Part model, mm, in its own coordinate system. A direction names the side the tool comes from. Coordinates: 2 decimals unless noted, no trailing zeros. Write each loop counter-clockwise with the first axis right and the second up, starting at its lowest first coordinate (ties: lowest second). Pieces come first, ordered by that corner, then holes. Notation, with made-up numbers: M 15,44 L 42,44 A4 ccw 42,51 Z; hole C 12.5,-8.5 d5. An arc over 180 degrees is marked long. Use a Markdown table: item, result. Add a question column.
Q1. Slice it at B-B on y = 22.5. Write the cut outline in (x, z).
Q2. Mould opens along Y. For faces 4 (the flat face through (1.5, 26, 14.8)), 5 (the flat face through (19, 10, 15)), 6 (the flat face through (-9, 23, 17)) say: released by +Y, released by -Y, zero draft, split by the parting line, or undercut.
Q3. Slice it at A-A on z = 18. Write the cut outline in (x, y), then the cut area to 3 significant figures.
Q4. Slice it at C-C on x = 1. Write the cut outline in (y, z), then the cut area to 3 significant figures.
Q5. Pin check, flat tips, straight feed: pin 1 Ø6 at (x, z) = (16.5, 10) entering from -Y; pin 2 Ø1.5 at (x, z) = (18, 10.5) entering from +Y; pin 3 Ø8 at (y, z) = (3.5, 8) entering from +X. Stop position of each tip, or through.
Q6. Slice it at D-D on x = -20.5. Write the cut outline in (y, z).
Q7. Wall check: L1, parallel to Z at x = -17.5, y = 19.75; L2, parallel to X at y = 3.5, z = 1; L3, parallel to Y at x = 2, z = 19. Give the ranges that are in metal, low to high. Write a range as from..to.
Q8. Tool access for faces 1 (the flat face through (13, 5, 15)), 2 (the flat face through (17, 24, 5)), 3 (the flat face through (-13, 5, 15)): list every direction of +Z, -Z, +X, -X, +Y, -Y with a clear straight run to the whole face (end or side of a thin tool).
from build123d import *

# Parameters (mm, degrees)
EXTRUDE_1_DEPTH = 30
SKETCH_2_W      = 50
SKETCH_2_H      = 20
EXTRUDE_2_DEPTH = 5


with BuildPart() as part:
    # Эскиз1 → Бобышка-Вытянуть1 (new body)
    with BuildSketch(Plane.XY):
        Polygon((9, 17), (9, 23.5), (3, 23.5), (0, 18.5), (0, 0), (13, 0), (13, 10), (25, 10), (25, 17), align=None)
        Polygon((3, 23.5), (9, 23.5), (9, 30), (0, 30), (0, 28.5), align=None)
    extrude_1 = extrude(amount=EXTRUDE_1_DEPTH)

    # Зеркальное отражение1: Бобышка-Вытянуть1 across plane
    add(extrude_1.mirror(Plane(origin=(0, 0, 30), x_dir=(0, 0, 1), z_dir=(-1, 0, 0))))

    # Эскиз2 → Бобышка-Вытянуть2 (add)
    with BuildSketch(Plane(origin=(0, 0, 0), x_dir=(-1, 0, 0), z_dir=(0, 0, -1))):
        with Locations((0, 20)):
            Rectangle(SKETCH_2_W, SKETCH_2_H)
        Polygon((0, 28.5), (3, 23.5), (0, 18.5), (-3, 23.5), align=None, mode=Mode.SUBTRACT)
    extrude(amount=-EXTRUDE_2_DEPTH)


solid = part.part
Recorded:
| question | item | result |
|---|---|---|
| 1 | outline | M -25,0 L -2.4,0 L -2.4,30 L -9,30 L -9,5 L -25,5 Z; M 2.4,0 L 25,0 L 25,5 L 9,5 L 9,30 L 2.4,30 Z |
| 2 | face 4 | undercut |
| 2 | face 5 | released by -Y |
| 2 | face 6 | zero draft |
| 3 | outline | M -25,10 L -13,10 L -13,0 L 13,0 L 13,10 L 25,10 L 25,17 L 9,17 L 9,30 L -9,30 L -9,17 L -25,17 Z; hole M -3,23.5 L 0,18.5 L 3,23.5 L 0,28.5 Z |
| 3 | area | 814 mm² |
| 4 | outline | M 0,0 L 20.17,0 L 20.17,30 L 0,30 Z; M 26.83,0 L 30,0 L 30,30 L 26.83,30 Z |
| 4 | area | 700 mm² |
| 5 | pin 1 | y = 10 |
| 5 | pin 2 | y = 17 |
| 5 | pin 3 | x = 13 |
| 6 | outline | M 10,0 L 30,0 L 30,5 L 17,5 L 17,30 L 10,30 Z |
| 7 | L1 | 0..5 |
| 7 | L2 | -13..13 |
| 7 | L3 | 0..21.83, 25.17..30 |
| 8 | face 1 | +Z, -Z, +X, -Y |
| 8 | face 2 | +Z, +X, +Y |
| 8 | face 3 | +Z, -Z, -X, -Y |
